Here's how the part is built. I have some questions about the finished solid (model axes, mm). A direction names the side the tool comes from. Coordinates: 2 decimals unless noted, no trailing zeros. Use CSV: the item, a comma, the result in double quotes. Start each with the question number.
```python
from build123d import *

# Parameters (mm, degrees)
F0_W      = 50.8
F0_H      = 57.15
F1_DEPTH  = 7.9375
F2_W      = 12.7
F2_H      = 69.85
F3_DEPTH  = 7.9375
F4_W      = 12.7
F4_H      = 69.85
F4_W_2    = 6.35
F5_DEPTH  = 1.5875
F6_W      = 50.8
F6_H      = 7.9375
F7_DEPTH  = 25.4
F7_TAPER  = 3
F8_W      = 80.01
F8_H      = 67.31
F9_DEPTH  = 3.175
F10_R     = 4.7625
F11_DEPTH = 9.525
F12_R     = 3.175
F13_DEPTH = 9.525


with BuildPart() as f1:
    # F0 (on Front) → F1 (new body)
    with BuildSketch(Plane.XZ):
        Polygon((0, 69.85), (0, 0), (82.55, 0), (82.55, 69.85), (69.85, 69.85), (19.05, 69.85), align=None)
        with Locations((44.45, 98.425)):
            Rectangle(F0_W, F0_H)
    extrude(amount=F1_DEPTH)

    # F2 (on face) → F3 (join)
    with BuildSketch(Plane(origin=(0, 0, 0), x_dir=(-1, 0, 0), z_dir=(0, 1, 0))):
        with Locations((-6.35, 34.925)):
            Rectangle(F2_W, F2_H)
        with Locations((-76.2, 34.925)):
            Rectangle(F2_W, F2_H)
    extrude(amount=F3_DEPTH)

    # F4 (on face) → F5 (join)
    with BuildSketch(Plane(origin=(0, 0, 0), x_dir=(-1, 0, 0), z_dir=(0, 1, 0))):
        with Locations((-19.05, 34.925)):
            Rectangle(F4_W, F4_H)
        with Locations((-66.675, 34.925)):
            Rectangle(F4_W_2, F4_H)
    extrude(amount=F5_DEPTH)

    # F6 (on face) → F7 (join)
    with BuildSketch(Plane(origin=(0, 0, 0), x_dir=(-1, 0, 0), z_dir=(0, 1, 0))):
        with Locations((-44.45, 123.03125)):
            Rectangle(F6_W, F6_H)
    extrude(amount=F7_DEPTH, taper=F7_TAPER)

    # F8 (on face) → F9 (join)
    with BuildSketch(Plane.XZ.offset(7.9375)):
        with Locations((41.275, 34.925)):
            Rectangle(F8_W, F8_H)
    extrude(amount=F9_DEPTH)

    # F10 (on face) → F11 (cut)
    with BuildSketch(Plane.XZ.offset(11.1125)):
        with Locations((15.875, 15.875)):
            Circle(F10_R)
        with Locations((66.675, 15.875)):
            Circle(F10_R)
    extrude(amount=-F11_DEPTH, mode=Mode.SUBTRACT)

    # F12 (on face) → F13 (cut)
    with BuildSketch(Plane(origin=(0, 7.9375, 0), x_dir=(-1, 0, 0), z_dir=(0, 1, 0))):
        with Locations((-76.2, 50.8)):
            Circle(F12_R)
        with Locations((-76.2, 19.05)):
            Circle(F12_R)
        with Locations((-6.35, 50.8)):
            Circle(F12_R)
        with Locations((-6.35, 19.05)):
            Circle(F12_R)
    extrude(amount=-F13_DEPTH, mode=Mode.SUBTRACT)


solid = f1.part
```
Item 1: I'm going to push flat-ended pins straight in: pin 1 (5 mm diameter, centred on x = 5.5, z = 51, fed in from +Y); pin 2 (10 mm diameter, centred on x = 19.5, z = 14, fed in from +Y); pin 3 (3.5 mm diameter, centred on x = 55.5, y = -9.5, fed in from -Z); pin 4 (5 mm diameter, centred on x = 6.35, z = 50.8, fed in from +Y). Where does each tip first touch, or does it pass through?
Item 2: Which directions (+Z, -Z, +X, -X, +Y, -Y) give clear straight access to the entire face, cutting with the end or side of a thin tool? Please do faces 4 (the flat face through (1.27, -10, 34)), 5 (the flat face through (41, -10, 68.58)), 6 (the flat face through (12.7, 5, 34)), 7 (the flat face through (76, -1.588, 51)).
Item 3: If I drill on line 1 along X through (y, z) = (5, 19); line 2 along X through (y, z) = (2.5, 58.5); line 3 along X through (y, z) = (1.5, 21.5), over which ranges is the centre line in solid material (lowest first)?
Item 4: Thinking about a two-plate mould opening in Z: for faces 1 (the flat face through (42, -2, 0)), 2 (the flat face through (0, 0, 34)), 3 (the cylindrical face through (7.04, 3.24, 15.95)), which applies, +Z half, -Z half, draft (parallel to the pull), parting line (faces both ways), or undercut?
Item 5: I want a section at A-A on y = -5. Count the separate pieces of the cut face and the enclosed holes in it, then the cut area to 3 significant figures.
Geometry says:
1,pin 1,"y = 7.94"
1,pin 2,"y = 1.59"
1,pin 3,"z = 0"
1,pin 4,"y = -1.59"
2,face 4,"+Z, -Z, -X, -Y"
2,face 5,"+Z, +X, -X, -Y"
2,face 6,"+Z, -Z, +Y"
2,face 7,"+Y"
3,line 1,"0 to 3.18, 9.52 to 12.7, 69.85 to 73.03, 79.37 to 82.55"
3,line 2,"0 to 12.7, 69.85 to 82.55"
3,line 3,"0 to 4.33, 8.37 to 25.4, 63.5 to 74.18, 78.22 to 82.55"
4,face 1,"-Z half"
4,face 2,"draft"
4,face 3,"undercut"
5,separate pieces,"1"
5,enclosed holes,"2"
5,area,"8,530 mm2"
